```python
from build123d import *

# Parameters (mm, degrees)
SKETCH1_R           = 16
BOSS_EXTRUDE1_DEPTH = 20


with BuildPart() as part:
    # Sketch1 → Boss-Extrude1 (new body)
    with BuildSketch(Plane.XY):
        Polygon((-40, -29), (-39, -30), (39, -30), (40, -29), (40, -6), (39, -5), (20.5, -5), (20.5, 17), (18.5, 19), (-18.5, 19), (-20.5, 17), (-20.5, -5), (-39, -5), (-40, -6), align=None)
        Circle(SKETCH1_R, mode=Mode.SUBTRACT)
    extrude(amount=-BOSS_EXTRUDE1_DEPTH)

    # Sketch2 → Cut-Revolve1 (revolve, cut)
    with BuildSketch(Plane.XY.offset(-10)):
        Polygon((30, -5), (35.5, -5), (34.5, -6), (34.5, -29), (35.5, -30), (30, -30), align=None)
    revolve(axis=Axis((30, -30, -10), (0, 1, 0)), mode=Mode.SUBTRACT)

    # Sketch3 → Cut-Revolve2 (revolve, cut)
    with BuildSketch(Plane.XY.offset(-10)):
        Polygon((-30, -5), (-24.5, -5), (-25.5, -6), (-25.5, -29), (-24.5, -30), (-30, -30), align=None)
    revolve(axis=Axis((-30, -30, -10), (0, 1, 0)), mode=Mode.SUBTRACT)


solid = part.part
```
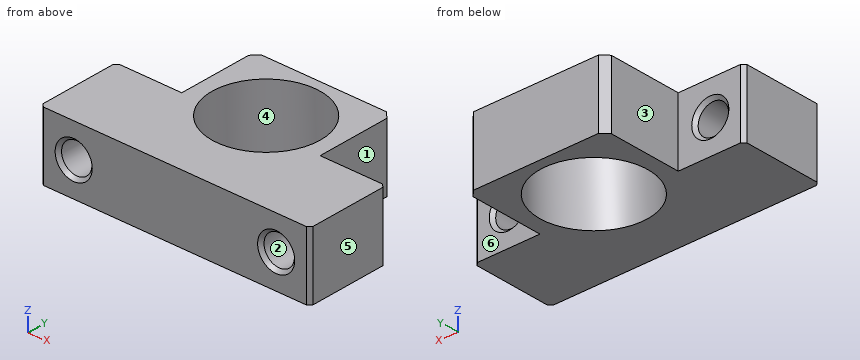
Check sheet for the modelled part. Datum: model origin and axes. Units: mm. Face numbers are marked on the shaded views. A direction names the side the tool comes from. Coordinates: 2 decimals unless noted, no trailing zeros. Loops run counter-clockwise (first coordinate to the right, second up) from the corner with the lowest first, then second, coordinate; pieces in that order, holes last. Notation, with made-up numbers: M 70.25,74.5 L 90.25,74.5 A18 cw 90.25,108.5 Z; hole C 77.25,23 d8. An arc over 180 degrees is marked long. Answer as a JSON object with one key per item and string values.
1. Release check for a two-part mould opening along Y. For the marked faces 4, 5 and 6 record: pulls with the +Y half, pulls with the -Y half, needs draft (parallel to the pull), parting line crosses it, or undercut.
Outcome:
{"face 4": "undercut", "face 5": "needs draft", "face 6": "pulls with the +Y half"}
2. Depth check by flat-ended pin: P1, Ø1, axis at y = 1, z = -9.5, coming from the +X side; P2, Ø5.5, axis at x = -30, z = -10, coming from the -Y side; P3, Ø11.5, axis at x = 30, z = -10, coming from the +Y side. Enter the tip coordinate at first touch or a pass-through.
Outcome:
{"P1": "x = 20.5", "P2": "through", "P3": "y = -5"}
3. Sectioned sample at C-C on y = -14.5. Record the cut outline in (x, z), and give its area (3 significant figures).
Outcome:
{"outline": "M -40,-20 L -6.76,-20 L -6.76,0 L -40,0 Z; M 6.76,-20 L 40,-20 L 40,0 L 6.76,0 Z; hole C -30,-10 d9; hole C 30,-10 d9", "area": "1,200 mm²"}
4. Sectioned sample at A-A on z = -10. Count the separate pieces of the cut face and the enclosed holes in it, and give its area (3 significant figures).
Outcome:
{"separate pieces": "3", "enclosed holes": "1", "area": "1,720 mm²"}
5. Sectioned sample at D-D on y = 0. Record the cut outline in (x, z).
Outcome:
{"outline": "M -20.5,-20 L -16,-20 L -16,0 L -20.5,0 Z; M 16,-20 L 20.5,-20 L 20.5,0 L 16,0 Z"}
6. Sectioned sample at B-B on x = 0. Record the cut outline in (y, z).
Outcome:
{"outline": "M -30,-20 L -16,-20 L -16,0 L -30,0 Z; M 16,-20 L 19,-20 L 19,0 L 16,0 Z"}
7. Access from +Z, -Z, +X, -X, +Y, -Y to the whole of each face (thin tool, end or side, straight path). Record for the marked faces 1, 2 and 3.
Outcome:
{"face 1": "+Z, -Z, +X, +Y", "face 2": "+Y, -Y", "face 3": "+Z, -Z, -X, +Y"}
8. Scan lines: L1, parallel to X at y = -21.5, z = -10; L2, parallel to Z at x = 30, y = -20.5; L3, parallel to X at y = -23, z = -13.5. Record each from-to range of solid material in increasing order. Write a range as from..to.
Outcome:
{"L1": "-40..-34.5, -25.5..25.5, 34.5..40", "L2": "-20..-14.5, -5.5..0", "L3": "-40..-32.83, -27.17..27.17, 32.83..40"}
